Could you check a few things on this model? Use its own coordinates, in mm. A direction names the side the tool comes from. Round coordinates to 2 decimals unless told otherwise and drop trailing zeros. Loops run counter-clockwise (first coordinate to the right, second up) from the corner with the lowest first, then second, coordinate; pieces in that order, holes last. Notation, with made-up numbers: (53.5, 73) -> (104.5, 73) arc R14 ccw to (104.5, 93) -> close; hole circle Ø10 at (63.25, -32.75). An arc over 180 degrees is marked (long way). Put each result on its own line as item: value. Start each with the question number.
1. Imagine slicing it at D-D, the plane y = 4.5. Please give me the cut outline in (x, z).
2. Which directions (+Z, -Z, +X, -X, +Y, -Y) give clear straight access to the entire face, cutting with the end or side of a thin tool? Please do faces 5 (the flat face through (-14, 3, 5)), 6 (the cylindrical face through (-9.46, -2.3, 3.73)).
3. I need wall thicknesses on line 1 (Z direction, x = -6.5, y = 13.5); line 2 (X direction, y = -1, z = 0.6); line 3 (Y direction, x = -17.5, z = 4.75). Which ranges of each line are inside material? Lowest first, please. Write a range as [from, to].
4. Imagine slicing it at A-A, the plane y = 0. Please give me the cut outline in (x, z), and give its area (3 significant figures).
5. If we mould it in two halves opening along Y, with no side actions, what happens to faces 1 (the cylindrical face through (-18, 0, 2)), 2 (the flat face through (0, 0, 2.5)), 3 (the cylindrical face through (-35, 0, 1)), 4 (the flat face through (0, -20, 1))? For each: pulls with the +Y half, pulls with the -Y half, needs draft (parallel to the pull), parting line crosses it, or undercut.
6. Imagine slicing it at B-B, the plane z = 1.15. Please give me the cut outline in (x, y).
7. Imagine slicing it at C-C, the plane z = 4.3. Please give me the cut outline in (x, y).
```python
from build123d import *

# Parameters (mm, degrees)
F0_R     = 6
F0_R_2   = 2
F1_DEPTH = 2.5
F0_R_3   = 3
F2_DEPTH = 5


with BuildPart() as f1:
    # F0 (on Top) → F1 (new body)
    with BuildSketch(Plane.XY):
        with BuildLine():
            Line((15, 20), (-15, 20))
            ThreePointArc((-15, 20), (-35, 0), (-15, -20))
            Line((-15, -20), (15, -20))
            ThreePointArc((15, -20), (35, 0), (15, 20))
        make_face()
        with Locations((-15, 0)):
            Circle(F0_R, mode=Mode.SUBTRACT)
        with Locations((15, 0)):
            Circle(F0_R_2, mode=Mode.SUBTRACT)
    extrude(amount=F1_DEPTH)

    # F0 (on Top) → F2 (join)
    with BuildSketch(Plane.XY):
        with Locations((-15, 0)):
            Circle(F0_R)
        with Locations((-15, 0)):
            Circle(F0_R_3, mode=Mode.SUBTRACT)
    extrude(amount=F2_DEPTH)


solid = f1.part
```
Entries:
1. outline: (-34.49, 0) -> (34.49, 0) -> (34.49, 2.5) -> (-11.03, 2.5) -> (-11.03, 5) -> (-18.97, 5) -> (-18.97, 2.5) -> (-34.49, 2.5) -> close
2. face 5: +Z, +X, -X, +Y, -Y
2. face 6: +Z
3. line 1: [0, 2.5]
3. line 2: [-34.97, -17.83], [-12.17, 13.27], [16.73, 34.97]
3. line 3: [-5.45, -1.66], [1.66, 5.45]
4. outline: (-35, 0) -> (-18, 0) -> (-18, 5) -> (-21, 5) -> (-21, 2.5) -> (-35, 2.5) -> close; (-12, 0) -> (13, 0) -> (13, 2.5) -> (-9, 2.5) -> (-9, 5) -> (-12, 5) -> close; (17, 0) -> (35, 0) -> (35, 2.5) -> (17, 2.5) -> close
4. area: 165 mm^2
5. face 1: undercut
5. face 2: needs draft
5. face 3: parting line crosses it
5. face 4: pulls with the -Y half
6. outline: (-15, -20) -> (15, -20) arc R20 ccw to (15, 20) -> (-15, 20) arc R20 ccw to start; hole circle Ø6 at (-15, 0); hole circle Ø4 at (15, 0)
7. outline: circle Ø12 at (-15, 0); hole circle Ø6 at (-15, 0)
